Autodesk Inventor part; units mm, degrees
ref_plane "Work Plane1" through (0, 101.6, 0) normal (0, 1, 0) x (-1, 0, 0)
ref_plane "YZ Plane" through (0, 0, 0) normal (1, 0, 0) x (0, 1, 0)
ref_plane "XY Plane" through (0, 0, 0) normal (0, 0, 1) x (1, 0, 0)
sketch "Sketch1" plane through (0, 0, 0) normal (0, 1, 0) x (-1, 0, 0)
  circle A0 centre (0, 0) radius 10.795
  circle A1 centre (0, 37.7825) radius 10.795
  dimension "d11" = 21.59
extrude "Extrusion1" add sketch "Sketch1" along normal blind 101.6 contours A0
sketch "Sketch2" plane through (0, 0, 0) normal (0, 1, 0) x (-1, 0, 0)
  circle A0 centre (0, 27.7858) radius 12.7
  point P0 (0, 0)
  dimension "d2" = 25.4
extrude "Extrusion2" add sketch "Sketch2" along normal blind 50.8
sketch "Sketch3" plane through (0, 0, 0) normal (0, 1, 0) x (-1, 0, 0)
  arc A0 (17.4625, 26.9867) -> (-17.4625, 28.5282) centre (-0.0401, 26.849) ccw
  arc A1 (-17.4625, 0) -> (17.4625, 0) centre (0, 0) ccw
  line L0 (17.4625, 0) -> (17.4625, 26.9867)
  line L1 (-17.4625, 0) -> (-17.4625, 28.5282)
extrude "Extrusion3" add sketch "Sketch3" against normal blind 10.16
sketch "Sketch4" plane through (0, 0, 0) normal (0, 1, 0) x (-1, 0, 0)
  point P0 (0, 0)
ref_plane "Work Plane1" through (0, 101.6, 0) normal (0, 1, 0) x (-1, 0, 0)
sketch "Sketch5" plane through (0, 101.6, 0) normal (0, 1, 0) x (-1, 0, 0)
  circle A0 centre (0, 0) radius 7.9375
  dimension "d8" = 15.875
extrude "Extrusion4" add sketch "Sketch5" along normal blind 101.6
sketch "Sketch6" plane through (0, 0, 0) normal (1, 0, 0) x (0, 1, 0)
  circle A0 centre (190.95, 0) radius 3.25
  line L0 (203.2, -7.9375) -> (203.2, 7.9375)
  line L1 (203.2, -7.9375) -> (203.2, 7.9375)
  point P0 (0, 0)
  dimension "d14" = 6.5
  dimension "d15" = 12.25
extrude "Extrusion5" cut sketch "Sketch6" along normal mid plane 101.6
properties part number "Linear Actuator"
Could you check a few things on this model? Use its own coordinates, in mm. A direction names the side the tool comes from. Round coordinates to 2 decimals unless told otherwise and drop trailing zeros. Loops run counter-clockwise (first coordinate to the right, second up) from the corner with the lowest first, then second, coordinate; pieces in that order, holes last. Notation, with made-up numbers: (53, 10) -> (102, 10) arc R29 ccw to (102, 30) -> close; hole circle Ø8 at (35.5, 18.25). An arc over 180 degrees is marked (long way). Use CSV: the item, a comma, the result in double quotes.
(1) Suppose I cut it at D-D on y = 11.5. Write out the boundary of the cut face in (x, z) (3 decimals).
Return value:
outline,"circle Ø25.4 at (0, 27.786); circle Ø21.59 at (0, 0)"
(2) If I drill on probe 1 along Y at (x, z) = (-1.5, 0); probe 2 along Y at (x, z) = (12, 20); probe 3 along Y at (x, z) = (-3, -10), over which ranges is the centre line in solid material (lowest first)? Write a range as [from, to].
Return value:
probe 1,"y = [-10.16, 187.7], [194.2, 203.2]"
probe 2,"y = [-10.16, 0]"
probe 3,"y = [-10.16, 101.6]"
(3) Suppose I cut it at B-B on z = -5.5. Write out the boundary of the cut face in (x, y), plus the area to 3 significant figures.
Return value:
outline,"(-16.57, -10.16) -> (16.57, -10.16) -> (16.57, 0) -> (9.29, 0) -> (9.29, 101.6) -> (5.72, 101.6) -> (5.72, 203.2) -> (-5.72, 203.2) -> (-5.72, 101.6) -> (-9.29, 101.6) -> (-9.29, 0) -> (-16.57, 0) -> close"
area,"3,390 mm²"
(4) Will these pins go through, and if not, where does the flat tip stop? pin 1 Ø10 at (x, y) = (-7.5, 89.5) entering from +Z; pin 2 Ø8 at (y, z) = (87.5, -6.5) entering from -X; pin 3 Ø12 at (x, y) = (6.5, 60.5) entering from +Z; pin 4 Ø5 at (x, y) = (-12.5, 140.5) entering from -Z.
Return value:
pin 1,"stops at z = 10.5"
pin 2,"stops at x = -10.5"
pin 3,"stops at z = 10.78"
pin 4,"passes through"
(5) Suppose I cut it at C-C on y = 109. Write out the boundary of the cut face in (x, z) (1 decimal), plus the area to 3 significant figures.
Return value:
outline,"circle Ø15.9 at (0, 0)"
area,"198 mm²"
(6) If we mould it in two halves opening along Z, with no side actions, what happens to faces 1 (the flat face through (0, 203.2, 0)), 2 (the cylindrical face through (7.956, 50.089, -7.296)), 3 (the cylindrical face through (0.38, -5.01, -17.46))? For each: +Z half, -Z half, draft (parallel to the pull), parting line (faces both ways), or undercut.
Return value:
face 1,"draft"
face 2,"undercut"
face 3,"-Z half"
(7) For faces 4 (the cylindrical face through (1.72, 151.69, 7.75)), 5 (the flat face through (0, -10.16, 14)), 6 (the flat face through (0, 50.8, 28)), which set-ups out of +Z, -Z, +X, -X, +Y, -Y let a thin tool reach every point of the face, with its end or its side?
Return value:
face 4,"+Y"
face 5,"+Z, -Z, +X, -X, -Y"
face 6,"+Z, +X, -X, +Y"
